Part model, mm, in its own coordinate system. A direction names the side the tool comes from. Give positions to 0.01 mm unless a question says otherwise; leave off trailing zeros. Write each loop counter-clockwise with the first axis right and the second up, starting at its lowest first coordinate (ties: lowest second). Pieces come first, ordered by that corner, then holes. Notation, with made-up numbers: M 3,23 L 43,23 A16 cw 43,40 Z; hole C -15.75,38.5 d11. An arc over 180 degrees is marked long. Answer as CSV lines item,"result". Start each with the question number.
1) Pin check, flat tips, straight feed: pin 1 Ø3 at (x, z) = (2, -3.5) entering from +Y; pin 2 Ø1.5 at (x, y) = (-2, 6.5) entering from -Z. Stop position of each tip, or through.
2) Slice it at B-B, the plane z = 1. Give the cut face in (x, y), plus the area to 3 significant figures.
3) Slice it at A-A, the plane x = 0. Give the cut face in (y, z).
4) Mould opens along Y. For faces 1 (the flat face through (-7.5, 0, 3)), 2 (the cylindrical face through (0, 1, 3)), 3 (the flat face through (0, -11.5, -2)) say: pulls with the +Y half, pulls with the -Y half, needs draft (parallel to the pull), parting line crosses it, or undercut.
5) Wall check: line 1 along Y through (x, z) = (0, 1.25); line 2 along Y through (x, z) = (-6.5, -1); line 3 along Z through (x, y) = (6.75, 11). Give the ranges that are in metal, low to high. Write a range as from..to.
6) Slice it at D-D, the plane x = -2.25. Give the cut face in (y, z).
7) Slice it at C-C, the plane y = -4.5. Give the cut face in (x, z), plus the area to 3 significant figures.
8) Tool access for faces 4 (the flat face through (-2, 2, 0)), 5 (the flat face through (0, 15.5, 3)): list every direction of +Z, -Z, +X, -X, +Y, -Y with a clear straight run to the whole face (end or side of a thin tool).
```python
from build123d import *

# Parameters (mm, degrees)
SKETCH1_W           = 15
SKETCH1_H           = 31
BOSS_EXTRUDE1_DEPTH = 6
SKETCH2_R           = 1.5
CUT_EXTRUDE1_DEPTH  = 6
SKETCH3_W           = 15
SKETCH3_H           = 4
BOSS_EXTRUDE2_DEPTH = 5


with BuildPart() as part:
    # Sketch1 → Boss-Extrude1 (new body)
    with BuildSketch(Plane.XY):
        Rectangle(SKETCH1_W, SKETCH1_H)
    extrude(amount=BOSS_EXTRUDE1_DEPTH)

    # Sketch2 → Cut-Extrude1 (cut)
    with BuildSketch(Plane.XY.offset(6)):
        with Locations((0, 9.5)):
            Circle(SKETCH2_R)
        with Locations((0, 2.5)):
            Circle(SKETCH2_R)
        with Locations((0, -4.5)):
            Circle(SKETCH2_R)
    extrude(amount=-CUT_EXTRUDE1_DEPTH, mode=Mode.SUBTRACT)

    # Sketch3 → Boss-Extrude2 (add)
    with BuildSketch(Plane(origin=(0, 0, 0), x_dir=(-1, 0, 0), z_dir=(0, 0, -1))):
        with Locations((0, -13.5)):
            Rectangle(SKETCH3_W, SKETCH3_H)
    extrude(amount=BOSS_EXTRUDE2_DEPTH)


solid = part.part
```
Found:
1,pin 1,"y = -11.5"
1,pin 2,"z = 0"
2,outline,"M -7.5,-15.5 L 7.5,-15.5 L 7.5,15.5 L -7.5,15.5 Z; hole C 0,-4.5 d3; hole C 0,2.5 d3; hole C 0,9.5 d3"
2,area,"444 mm²"
3,outline,"M -15.5,-5 L -11.5,-5 L -11.5,0 L -6,0 L -6,6 L -15.5,6 Z; M -3,0 L 1,0 L 1,6 L -3,6 Z; M 4,0 L 8,0 L 8,6 L 4,6 Z; M 11,0 L 15.5,0 L 15.5,6 L 11,6 Z"
4,face 1,"needs draft"
4,face 2,"undercut"
4,face 3,"pulls with the +Y half"
5,line 1,"-15.5..-6, -3..1, 4..8, 11..15.5"
5,line 2,"-15.5..-11.5"
5,line 3,"0..6"
6,outline,"M -15.5,-5 L -11.5,-5 L -11.5,0 L 15.5,0 L 15.5,6 L -15.5,6 Z"
7,outline,"M -7.5,0 L -1.5,0 L -1.5,6 L -7.5,6 Z; M 1.5,0 L 7.5,0 L 7.5,6 L 1.5,6 Z"
7,area,"72.0 mm²"
8,face 4,"-Z, +X, -X, +Y"
8,face 5,"+Z, -Z, +X, -X, +Y"
